Geometry check sheet. Reference: the model listing, model coordinates, mm. A direction names the side the tool comes from. Round coordinates to 2 decimals unless told otherwise and drop trailing zeros. Order: outer loops, then holes, each group sorted by start corner. A loop starts at its lowest first (then second) coordinate and runs counter-clockwise, first axis right, second up.
(1) Sectioned sample at D-D (x = 192). Record the boundary of the cut face in (y, z).
(2) Material ranges on line 1 along Z through (x, y) = (124.5, 27); line 2 along X through (y, z) = (33.5, -109); line 3 along X through (y, z) = (6.5, -0.5), recorded low to high.
(3) Sectioned sample at B-B (y = 20). Record the boundary of the cut face in (x, z).
(4) Release check for a two-part mould opening along X. For faces 6 (the face through (59, 32.4, -14)), 7 (the face through (188.33, 14, 47)), 8 (the face through (66.87, 17, 47)) record: +X half, -X half, draft (parallel to the pull), parting line (faces both ways), or undercut.
(5) Set-up check for faces 1 (the face through (187, 35.4, 14)), 2 (the face through (63.87, 14, 43)), 3 (the face through (185.33, 17, 43)), 4 (the face through (127, 14, -121.747)), 5 (the face through (125, 14, 211.873)): record each of +Z, -Z, +X, -X, +Y, -Y from which the full face is reachable in a straight line by a thin tool's end or side.
(6) Sectioned sample at C-C (z = -0.5). Record the boundary of the cut face in (x, y), plus the area to 3 significant figures.
(7) Go/stop test with flat-tipped pins: pin 1 (17.5 mm diameter, centred on x = 107, y = 12, fed in from +Z); pin 2 (0.9 mm diameter, centred on x = 128, y = 34.5, fed in from -Z); pin 3 (17.5 mm diameter, centred on y = 11.5, z = 12, fed in from +X). Record where each tip stops, or that it passes through.
(8) Sectioned sample at A-A (x = 139). Record the boundary of the cut face in (y, z).
from build123d import *

# Parameters (mm, degrees)
BASE_FLANGE1_DEPTH  = 3
BOSS_EXTRUDE1_DEPTH = 35.4
BOSS_EXTRUDE2_DEPTH = 3


# Sheet-metal steps are written as plain solids
with BuildPart() as part:
    # Sketch1 → Base-Flange1 (new body)
    with BuildSketch(Plane(origin=(0, 0, 0), x_dir=(1, 0, 0), z_dir=(0, 1, 0))):
        Polygon((63.869646018, 121.746556797), (63.869646018, -211.873486949), (188.329646018, -211.873486949), (188.329646018, 121.746556797), (164.199646018, 121.746556797), (87.999646018, 121.746556797), align=None)
    extrude(amount=-BASE_FLANGE1_DEPTH)

    # Sketch75 → Boss-Extrude1 (add)
    with BuildSketch(Plane(origin=(0, 0, 0), x_dir=(1, 0, 0), z_dir=(0, 1, 0))):
        Polygon((188.329646018, -193.287020835), (188.329646018, 121.746556797), (185.329646018, 121.746556797), (164.199646018, 121.746556797), (87.999646018, 121.746556797), (63.869646018, 121.746556797), (63.869646018, -211.873486949), (66.869646018, -211.873486949), (188.329646018, -211.873486949), align=None)
        Polygon((167.199646018, 118.746556797), (185.329646018, 118.746556797), (185.329646018, -208.873486949), (66.869646018, -208.873486949), (66.869646018, 118.746556797), (84.999646018, 118.746556797), (87.999646018, 118.746556797), (164.199646018, 118.746556797), align=None, mode=Mode.SUBTRACT)
    extrude(amount=BOSS_EXTRUDE1_DEPTH)

    # Sketch76 → Boss-Extrude2 (add)
    with BuildSketch(Plane(origin=(0, 35.4, 0), x_dir=(1, 0, 0), z_dir=(0, 1, 0))):
        Polygon((188.329646018, 160.232979165), (168.60717256, 160.232979165), (158.199646018, 160.232979165), (158.199646018, 126.246556797), (93.999646018, 126.246556797), (93.999646018, 154.232979165), (93.999646018, 160.232979165), (61.173757876, 160.232979165), (50.869646018, 160.232979165), (50.869646018, -212.840780944), (50.869646018, -217.873486949), (190.329646018, -217.873486949), (201.329646018, -217.873486949), (201.329646018, 160.232979165), align=None)
        Polygon((63.869646018, -211.873486949), (63.869646018, 121.746556797), (87.999646018, 121.746556797), (142.998933393, 121.746556797), (164.199646018, 121.746556797), (188.329646018, 121.746556797), (188.329646018, -211.873486949), align=None, mode=Mode.SUBTRACT)
    extrude(amount=-BOSS_EXTRUDE2_DEPTH)


solid = part.part
Answer below:
1. outline: (32.4, -160.23) - (35.4, -160.23) - (35.4, 217.87) - (32.4, 217.87) - close
2. line 1: z = -121.75 to -118.75, 208.87 to 211.87
2. line 2: x = 50.87 to 66.87, 185.33 to 201.33
2. line 3: x = 63.87 to 66.87, 185.33 to 188.33
3. outline: (63.87, -121.75) - (188.33, -121.75) - (188.33, 211.87) - (63.87, 211.87) - close; hole (66.87, -118.75) - (185.33, -118.75) - (185.33, 208.87) - (66.87, 208.87) - close
4. face 6: draft
4. face 7: +X half
4. face 8: undercut
5. face 1: +Z, -Z, +X, -X, +Y
5. face 2: +Z, -Z, -X, -Y
5. face 3: +Y
5. face 4: -Z, +X, -X, -Y
5. face 5: +Z, +X, -X, -Y
6. outline: (50.87, 32.4) - (63.87, 32.4) - (63.87, -3) - (188.33, -3) - (188.33, 32.4) - (201.33, 32.4) - (201.33, 35.4) - (185.33, 35.4) - (185.33, 0) - (66.87, 0) - (66.87, 35.4) - (50.87, 35.4) - close
6. area: 664 mm2
7. pin 1: stops at z = 211.87
7. pin 2: stops at z = -126.25
7. pin 3: stops at x = 188.33
8. outline: (-3, -121.75) - (32.4, -121.75) - (32.4, -126.25) - (35.4, -126.25) - (35.4, -118.75) - (0, -118.75) - (0, 208.87) - (35.4, 208.87) - (35.4, 217.87) - (32.4, 217.87) - (32.4, 211.87) - (-3, 211.87) - close
